```python
from build123d import *

# Parameters (mm, degrees)
SKETCH1_R           = 25
BOSS_EXTRUDE1_DEPTH = 50
SKETCH2_R           = 17.5
CUT_EXTRUDE1_DEPTH  = 3
CUT_EXTRUDE2_START  = -3
SKETCH3_R           = 17.5
CUT_EXTRUDE2_DEPTH  = 3
SKETCH4_R           = 20
BOSS_EXTRUDE2_DEPTH = 60
SKETCH5_R           = 17.5
BOSS_EXTRUDE3_DEPTH = 3
FILLET1_R           = 3
FILLET2_R           = 2


with BuildPart() as part:
    # Sketch1 → Boss-Extrude1 (new body)
    with BuildSketch(Plane.XY):
        Circle(SKETCH1_R)
    extrude(amount=BOSS_EXTRUDE1_DEPTH)

    # Sketch2 → Cut-Extrude1 (cut)
    with BuildSketch(Plane.XY.offset(50)):
        Circle(SKETCH2_R)
    extrude(amount=-CUT_EXTRUDE1_DEPTH, mode=Mode.SUBTRACT)

    # Sketch3 → Cut-Extrude2 (cut)
    with BuildSketch(Plane(origin=(0, 0, 0), x_dir=(-1, 0, 0), z_dir=(0, 0, -1)).offset(CUT_EXTRUDE2_START)):
        with Locations(Location((0, 0, 0), (0, 0, 180))):
            Circle(SKETCH3_R)
    extrude(amount=CUT_EXTRUDE2_DEPTH, mode=Mode.SUBTRACT)

    # Sketch4 → Boss-Extrude2 (add)
    with BuildSketch(Plane(origin=(0, 0, 0), x_dir=(0, 0, -1), z_dir=(1, 0, 0))):
        with Locations((-25, 0)):
            Circle(SKETCH4_R)
    extrude(amount=BOSS_EXTRUDE2_DEPTH)

    # Sketch5 → Boss-Extrude3 (add)
    with BuildSketch(Plane(origin=(60, 0, 0), x_dir=(0, 0, -1), z_dir=(1, 0, 0))):
        with Locations((-25, 0)):
            Circle(SKETCH5_R)
    extrude(amount=BOSS_EXTRUDE3_DEPTH)

    # Fillet1
    fillet1_edges = [part.edges().sort_by_distance(p)[0] for p in [
        (15, 20, 25),
    ]]
    fillet(fillet1_edges, radius=FILLET1_R)

    # Fillet2
    fillet2_edges = [part.edges().sort_by_distance(p)[0] for p in [
        (-25, 0, 0),
        (-25, 0, 50),
    ]]
    fillet(fillet2_edges, radius=FILLET2_R - 0.0001)  # a hair under: the kernel refuses the full size


solid = part.part
```
For this review, take the finished solid that the model builds, in its own axes (mm). A direction names the side the tool comes from. Give positions to 0.01 mm unless a question says otherwise; leave off trailing zeros. Write each loop counter-clockwise with the first axis right and the second up, starting at its lowest first coordinate (ties: lowest second). Pieces come first, ordered by that corner, then holes. Notation, with made-up numbers: M 55.25,-30 L 77.25,-30 A17 cw 77.25,2 Z; hole C 86.5,68.25 d3. An arc over 180 degrees is marked long. Answer as CSV lines item,"result".
1. Wall thickness on line 1 (Z direction, x = -4, y = -5); line 2 (Y direction, x = 0, z = 46); line 3 (Y direction, x = 0, z = 49.45): over which ranges is each line inside the solid? List them lowest first.
Findings:
line 1,"z = 3 to 47"
line 2,"y = -25 to 25"
line 3,"y = -24.38 to -17.5, 17.5 to 24.38"
2. Consider section A-A, the plane x = 0. Write out the cut boundary in (y, z), then the cut area to 3 significant figures.
Findings:
outline,"M -25,2 A2 ccw -23,0 L -17.5,0 L -17.5,3 L 17.5,3 L 17.5,0 L 23,0 A2 ccw 25,2 L 25,48 A2 ccw 23,50 L 17.5,50 L 17.5,47 L -17.5,47 L -17.5,50 L -23,50 A2 ccw -25,48 Z"
area,"2,290 mm2"
3. For pin 1 (12 mm diameter, centred on x = -11.5, z = 30.5, fed in from -Y); pin 2 (12 mm diameter, centred on x = 10, y = 11.5, fed in from +Z); pin 3 (6 mm diameter, centred on x = 5.5, y = 8, fed in from +Z); pin 4 (8 mm diameter, centred on x = 28, y = -9, fed in from +Z), all flat-tipped, find the tip position at first contact; note any pin that passes through.
Findings:
pin 1,"stops at y = -24.39"
pin 2,"stops at z = 50"
pin 3,"stops at z = 47"
pin 4,"stops at z = 44.89"
4. Draft analysis for pull direction X (two halves, no side actions). For faces 5 (the flat face through (60, -18, 25)), 6 (the flat face through (0, 0, 47)), 7 (the cylindrical face through (61.479, -10.648, 38.887)), state which applies: +X half, -X half, draft (parallel to the pull), parting line (faces both ways), or undercut.
Findings:
face 5,"+X half"
face 6,"undercut"
face 7,"draft"
5. Consider section B-B, the plane x = 48. Write out the cut boundary in (y, z), then the cut area to 3 significant figures.
Findings:
outline,"C 0,25 d40"
area,"1,260 mm2"
6. For faces 1 (the flat face through (-8.63, 15.44, 0)), 2 (the cylindrical face through (-13.887, -10.648, 48.521)), 3 (the cylindrical face through (-3.794, 17.084, 1.521)), 4 (the cylindrical face through (42.568, 6.007, 5.924)), list the 3-axis set-ups (+Z, -Z, +X, -X, +Y, -Y) from which the entire face can be reached by the end or side of a thin tool; tool diameter is ignored.
Findings:
face 1,"-Z, +X, -X, +Y, -Y"
face 2,"+Z"
face 3,"-Z"
face 4,"+X"
